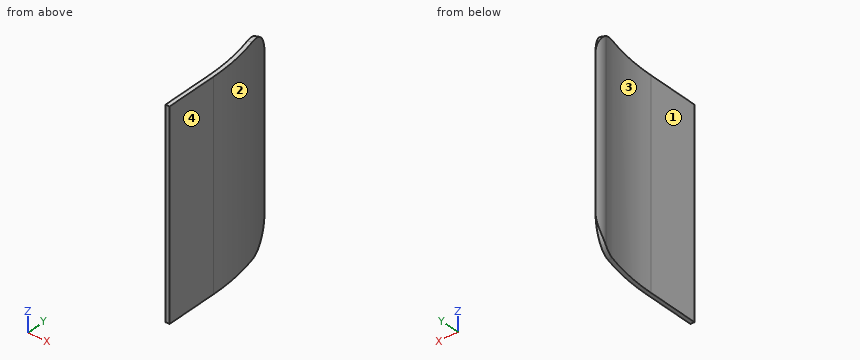
```python
from build123d import *

# Parameters (mm, degrees)
BOSS_EXTRUDE1_DEPTH = 375
FILLET1_R           = 100
FILLET2_R           = 100


with BuildPart() as part:
    # Sketch2 → Boss-Extrude1 (new, symmetric)
    with BuildSketch(Plane.XY):
        with BuildLine():
            Line((0, 0), (0, 197.03652177061554))
            ThreePointArc((0, 197.03652177061554), (-15.037794104979639, 351.42024926941554), (-59.58583829105939, 499.99999999999994))
            Line((-59.58583829105939, 499.99999999999994), (-45.68004275536319, 505.62395328211494))
            ThreePointArc((-45.68004275536319, 505.62395328211494), (-0.31663526116813046, 355.79479163998155), (15, 200))
            Line((15, 200), (15, 0))
            Line((15, 0), (0, 0))
        make_face()
    extrude(amount=BOSS_EXTRUDE1_DEPTH, both=True)

    # Fillet1
    fillet1_edges = [part.edges().sort_by_distance(p)[0] for p in [
        (-52.63294052321129, 502.8119766410574, 375),
        (-52.63294052321129, 502.8119766410574, -375),
    ]]
    fillet(fillet1_edges, radius=FILLET1_R)

    # Fillet2
    # the kernel refuses this fillet: 100 mm, written as the material it takes off along each edge
    with BuildSketch(Plane(origin=(-59.585838291059304, 500, -398.16540938759147), x_dir=(0.35002683735088513, -0.9367396720189324, 0), z_dir=(0, 0, 1))) as fillet2_piece_1:
        with BuildLine():
            CenterArc((52.34529898972619, 99.95258338935764), FILLET2_R, 238.16595036799683, 30.069556200548902)
            Line((-0.40077852073035836, 14.99464493001819), (-1.4557000709394878, 13.295486160831398))
            ThreePointArc((-1.4557000709394878, 13.295486160831398), (-2.1996752510342628, 7.443885328911702), (-1.9992859906690836, -0.05343713609739175))
            Line((-1.9992859906690836, -0.05343713609739175), (0.06158270469381519, -1.9990516677871575))
            ThreePointArc((0.06158270469381519, -1.9990516677871575), (24.633081877518478, -1.6206671148610328), (49.20458105034301, -1.999051667787162))
            Line((49.20458105034301, -1.999051667787162), (49.266163755036786, -3.27e-15))
        make_face()
    extrude(amount=796.3308187751829, mode=Mode.SUBTRACT)


solid = part.part
```
For this review, take the finished solid that the model builds, in its own axes (mm). Face numbers are marked on the shaded views. A direction names the side the tool comes from. Coordinates: 2 decimals unless noted, no trailing zeros. Write each loop counter-clockwise with the first axis right and the second up, starting at its lowest first coordinate (ties: lowest second). Pieces come first, ordered by that corner, then holes. Notation, with made-up numbers: (34.5, 25) - (39.5, 25) arc R26 ccw to (39.5, 57) - close; hole circle Ø9 at (73.25, 8.5). An arc over 180 degrees is marked (long way). Put each result on its own line as item: value.
1. Wall thickness on probe 1 along X at (y, z) = (150, -318); probe 2 along X at (y, z) = (418, -317.5): over which ranges is each line inside the solid? List them lowest first.
Values found:
probe 1: 0 to 15
probe 2: -31.12 to -15.28
2. For pin 1 (4 mm diameter, centred on y = 73.5, z = 65, fed in from -X); pin 2 (10 mm diameter, centred on y = 339.5, z = 168, fed in from -X); pin 3 (6 mm diameter, centred on y = 418, z = 141.5, fed in from +X), all flat-tipped, find the tip position at first contact; note any pin that passes through.
Values found:
pin 1: x = 0
pin 2: x = -13.71
pin 3: x = -14.43
3. Machinability: for the marked faces 1 and 2, which of the approach directions +Z, -Z, +X, -X, +Y, -Y give a long, thin tool a straight path to every point of the face, cutting with its end or side? Answer none if there is none.
Values found:
face 1: +Z, -Z, -X, -Y
face 2: +Z, -Z, +X, +Y
4. Add section A-A, the plane z = 100.5. Give the boundary of the cut face in (x, y).
Values found:
outline: (-45.68, 505.62) arc R100 ccw to (-42.34, 453.85) arc R800 cw to (0, 197.04) - (0, 0) - (15, 0) - (15, 200) arc R800 ccw to start
5. Mouldability with a two-part tool opening along X and no side actions: class the marked faces 3 and 4 as released by +X, released by -X, zero draft, split by the parting line, or undercut.
Values found:
face 3: released by -X
face 4: released by +X
6. Add section B-B, the plane y = 179.5. Give the boundary of the cut face in (x, z).
Values found:
outline: (0, -375) - (15, -375) - (15, 375) - (0, 375) - close
